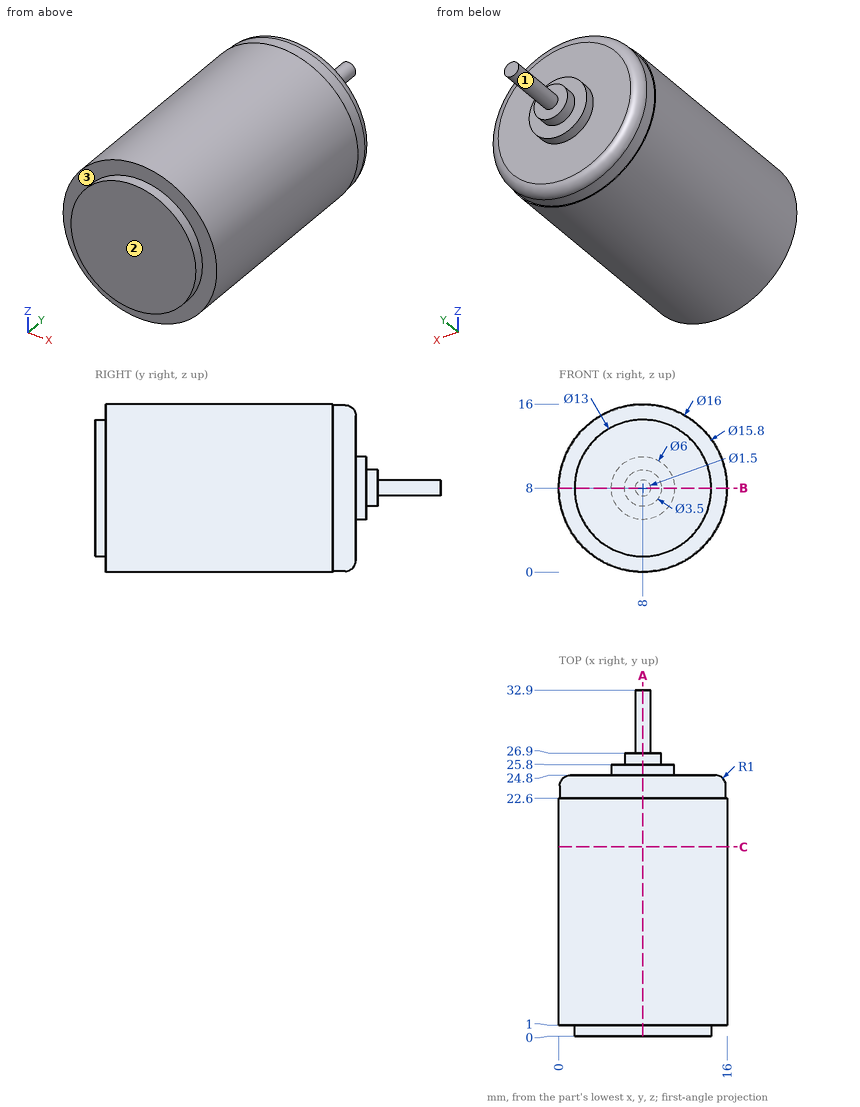
Check sheet for the drawn part. Datum: minimum x, y, z corner. Units: mm. A direction names the side the tool comes from. Coordinates: 2 decimals unless noted, no trailing zeros. Loops run counter-clockwise (first coordinate to the right, second up) from the corner with the lowest first, then second, coordinate; pieces in that order, holes last. Notation, with made-up numbers: (8, -33) -> (55, -33) arc R10 cw to (55, -21) -> close; hole circle Ø8 at (-13, -19). An arc over 180 degrees is marked (long way). Answer in a Markdown table with one row per item.
1. Sectioned sample at B-B, the plane z = 8. Record the boundary of the cut face in (x, y).
Check values:
| item | result |
|---|---|
| outline | (0, 1) -> (1.5, 1) -> (1.5, 0) -> (14.5, 0) -> (14.5, 1) -> (16, 1) -> (16, 22.6) -> (15.9, 22.6) -> (15.9, 23.8) arc R1 ccw to (14.9, 24.8) -> (11, 24.8) -> (11, 25.8) -> (9.75, 25.8) -> (9.75, 26.9) -> (8.75, 26.9) -> (8.75, 32.9) -> (7.25, 32.9) -> (7.25, 26.9) -> (6.25, 26.9) -> (6.25, 25.8) -> (5, 25.8) -> (5, 24.8) -> (1.1, 24.8) arc R1 ccw to (0.1, 23.8) -> (0.1, 22.6) -> (0, 22.6) -> close |
2. Access from +Z, -Z, +X, -X, +Y, -Y to the whole of each face (thin tool, end or side, straight path). Record for the marked faces 1, 2 and 3.
Check values:
| item | result |
|---|---|
| face 1 | +Y |
| face 2 | +Z, -Z, +X, -X, -Y |
| face 3 | -Y |
3. Sectioned sample at A-A, the plane x = 8. Record the boundary of the cut face in (y, z), then the cut area to 3 significant figures.
Check values:
| item | result |
|---|---|
| outline | (0, 1.5) -> (1, 1.5) -> (1, 0) -> (22.6, 0) -> (22.6, 0.1) -> (23.8, 0.1) arc R1 ccw to (24.8, 1.1) -> (24.8, 5) -> (25.8, 5) -> (25.8, 6.25) -> (26.9, 6.25) -> (26.9, 7.25) -> (32.9, 7.25) -> (32.9, 8.75) -> (26.9, 8.75) -> (26.9, 9.75) -> (25.8, 9.75) -> (25.8, 11) -> (24.8, 11) -> (24.8, 14.9) arc R1 ccw to (23.8, 15.9) -> (22.6, 15.9) -> (22.6, 16) -> (1, 16) -> (1, 14.5) -> (0, 14.5) -> close |
| area | 412 mm2 |
4. Sectioned sample at C-C, the plane y = 18. Record the boundary of the cut face in (x, z).
Check values:
| item | result |
|---|---|
| outline | circle Ø16 at (8, 8) |
5. Material ranges on line 1 along Y through (x, z) = (13, 8.75); line 2 along Y through (x, z) = (6, 7); line 3 along X through (y, z) = (2, 9.25), recorded low to high. Write a range as [from, to].
Check values:
| item | result |
|---|---|
| line 1 | y = [0, 24.8] |
| line 2 | y = [0, 25.8] |
| line 3 | x = [0.1, 15.9] |
6. Go/stop test with flat-tipped pins: pin 1 (3 mm diameter, centred on x = 14.5, y = 20, fed in from -Z) (3 decimals); pin 2 (2 mm diameter, centred on y = 3.5, z = 5.5, fed in from +X). Record where each tip stops, or that it passes through.
Check values:
| item | result |
|---|---|
| pin 1 | stops at z = 1.755 |
| pin 2 | stops at x = 15.86 |
